Check sheet for the modelled part. Datum: model origin and axes. Units: mm. Round coordinates to 2 decimals unless told otherwise and drop trailing zeros. Loops run counter-clockwise (first coordinate to the right, second up) from the corner with the lowest first, then second, coordinate; pieces in that order, holes last. Notation, with made-up numbers: (-10.5, 64.25) - (20.5, 64.25) arc R16 ccw to (20.5, 89.25) - close; hole circle Ø7 at (55, 22). An arc over 180 degrees is marked (long way). Put each result on its own line as item: value. Start each with the question number.
```python
from build123d import *

# Parameters (mm, degrees)
SKETCH1_W           = 69
SKETCH1_H           = 15
SKETCH1_R           = 3.05
SKETCH1_R_2         = 1.75
BOSS_EXTRUDE1_DEPTH = 8


with BuildPart() as part:
    # Sketch1 → Boss-Extrude1 (new body)
    with BuildSketch(Plane.XY):
        Rectangle(SKETCH1_W, SKETCH1_H)
        with Locations((-27, 0)):
            Circle(SKETCH1_R, mode=Mode.SUBTRACT)
        with Locations(Location((27, 0, 0), (0, 0, 180))):
            Circle(SKETCH1_R, mode=Mode.SUBTRACT)
        with Locations((0.25, 3.55)):
            Circle(SKETCH1_R_2, mode=Mode.SUBTRACT)
        with Locations((9.75, 3.55)):
            Circle(SKETCH1_R_2, mode=Mode.SUBTRACT)
    extrude(amount=BOSS_EXTRUDE1_DEPTH)


solid = part.part
```
Q1. Cross-section at A-A on x = 0.25. Enter the section's corners in (y, z), and give its area (3 significant figures).
Q2. Material ranges on line 1 (X direction, y = 3.75, z = 4.75); line 2 (Y direction, x = -27, z = 4.5); line 3 (X direction, y = 4.75, z = 2.75), recorded low to high. Write a range as from..to.
Q3. Cross-section at C-C on y = -2. Enter the section's corners in (x, z).
Q4. Cross-section at D-D on x = -27. Enter the section's corners in (y, z).
Q5. Cross-section at B-B on z = 1.5. Enter the section's corners in (x, y), and give its area (3 significant figures).
Q6. Draft check along X on faces 1 (the face through (-34.5, 0, 4)), 2 (the face through (0, -7.5, 4)), 3 (the face through (24.183, 1.168, 3.944)). Enter one of: +X half, -X half, draft (parallel to the pull), parting line (faces both ways), or undercut.
Answer list:
1. outline: (-7.5, 0) - (1.8, 0) - (1.8, 8) - (-7.5, 8) - close; (5.3, 0) - (7.5, 0) - (7.5, 8) - (5.3, 8) - close
1. area: 92.0 mm2
2. line 1: x = -34.5..-1.49, 1.99..8.01, 11.49..34.5
2. line 2: y = -7.5..-3.05, 3.05..7.5
2. line 3: x = -34.5..-1.02, 1.52..8.48, 11.02..34.5
3. outline: (-34.5, 0) - (-29.3, 0) - (-29.3, 8) - (-34.5, 8) - close; (-24.7, 0) - (24.7, 0) - (24.7, 8) - (-24.7, 8) - close; (29.3, 0) - (34.5, 0) - (34.5, 8) - (29.3, 8) - close
4. outline: (-7.5, 0) - (-3.05, 0) - (-3.05, 8) - (-7.5, 8) - close; (3.05, 0) - (7.5, 0) - (7.5, 8) - (3.05, 8) - close
5. outline: (-34.5, -7.5) - (34.5, -7.5) - (34.5, 7.5) - (-34.5, 7.5) - close; hole circle Ø6.1 at (-27, 0); hole circle Ø3.5 at (0.25, 3.55); hole circle Ø3.5 at (9.75, 3.55); hole circle Ø6.1 at (27, 0)
5. area: 957 mm2
6. face 1: -X half
6. face 2: draft
6. face 3: undercut
